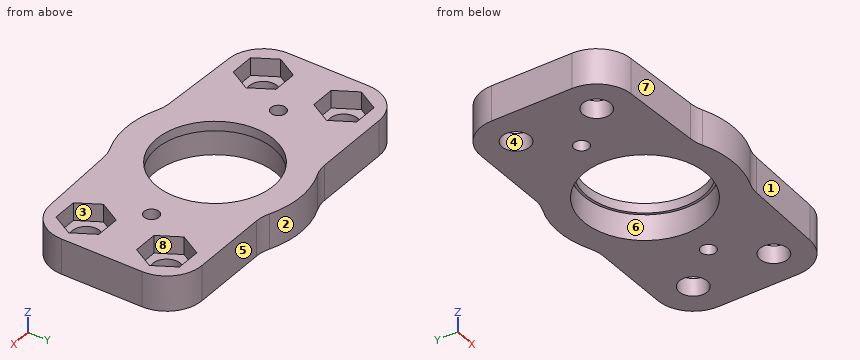
```python
from build123d import *

# Parameters (mm, degrees)
SKETCH_1_R          = 12.1
EXTRUDE_1_DEPTH     = 7
FILLET_3_R          = 7
SKETCH_7_R          = 12.1
SKETCH_7_R_2        = 11.6
EXTRUDE_2_DEPTH     = 1.9
HOLE_WIZARD_M53_D   = 5.5
HOLE_WIZARD_M54_D   = 5.5
CUT_EXTRUDE_1_DEPTH = 3.5
SKETCH1_R           = 1.475614807
CUT_EXTRUDE1_DEPTH  = 10


with BuildPart() as part:
    # Эскиз1 → Бобышка-Вытянуть1 (new body)
    with BuildSketch(Plane.XY):
        with BuildLine():
            Line((-9.282257481, -15.602398743), (-25.265839773, -14.994950265))
            ThreePointArc((-25.265839773, -14.994950265), (-30.042860221, -12.854849204), (-32, -8))
            Line((-32, -8), (-32, 15))
            Line((-32, 15), (-8, 15))
            ThreePointArc((-8, 15), (0, 17), (8, 15))
            Line((8, 15), (32, 15))
            Line((32, 15), (32, -8))
            ThreePointArc((32, -8), (30.042860221, -12.854849204), (25.265839773, -14.994950265))
            Line((25.265839773, -14.994950265), (9.282257481, -15.602398743))
            ThreePointArc((9.282257481, -15.602398743), (7.964469385, -15.770214084), (6.696960066, -16.167891819))
            ThreePointArc((6.696960066, -16.167891819), (0, -17.5), (-6.696960066, -16.167891819))
            ThreePointArc((-6.696960066, -16.167891819), (-7.964469385, -15.770214084), (-9.282257481, -15.602398743))
        make_face()
        Circle(SKETCH_1_R, mode=Mode.SUBTRACT)
    extrude(amount=EXTRUDE_1_DEPTH)

    # Скругление3
    fillet_3_edges = [part.edges().sort_by_distance(p)[0] for p in [
        (-32, 15, 3.5),
        (-8, 15, 3.5),
        (8, 15, 3.5),
        (32, 15, 3.5),
    ]]
    fillet(fillet_3_edges, radius=FILLET_3_R)

    # Эскиз7 → Бобышка-Вытянуть2 (add)
    with BuildSketch(Plane.XY.offset(7)):
        Circle(SKETCH_7_R)
        Circle(SKETCH_7_R_2, mode=Mode.SUBTRACT)
    extrude(amount=-EXTRUDE_2_DEPTH)

    # Отверстие с зазором M53 (through all)
    with Locations(Plane.XY.offset(7)):
        with Locations((-25, 8), (25, 8)):
            Hole(HOLE_WIZARD_M53_D / 2)

    # Отверстие с зазором M54 (through all)
    with Locations(Plane(origin=(-20.850360387, 7.199740636, 7), x_dir=(-1, 0, 0), z_dir=(0, 0, 1))):
        with Locations((-45.850360387, 15.199740636), (4.149639613, 15.199740636)):
            Hole(HOLE_WIZARD_M54_D / 2)

    # Эскиз18 → Вырез-Вытянуть1 (cut)
    with BuildSketch(Plane(origin=(0, 0, 7), x_dir=(1, 0, 0), z_dir=(0, 0, -1))):
        Polygon((20.092522712, -8), (22.546261356, -12.25), (27.453738644, -12.25), (29.907477288, -8), (27.453738644, -3.75), (22.546261356, -3.75), align=None)
        Polygon((-27.453738644, -3.75), (-29.907477288, -8), (-27.453738644, -12.25), (-22.546261356, -12.25), (-20.092522712, -8), (-22.546261356, -3.75), align=None)
        Polygon((20.092522712, 8), (22.546261356, 12.25), (27.453738644, 12.25), (29.907477288, 8), (27.453738644, 3.75), (22.546261356, 3.75), align=None)
        Polygon((-22.546261356, 12.25), (-20.092522712, 8), (-22.546261356, 3.75), (-27.453738644, 3.75), (-29.907477288, 8), (-27.453738644, 12.25), align=None)
    extrude(amount=CUT_EXTRUDE_1_DEPTH, mode=Mode.SUBTRACT)

    # Sketch1 → Cut-Extrude1 (cut)
    with BuildSketch(Plane.XY):
        with Locations((17.9, 0)):
            Circle(SKETCH1_R)
        with Locations((-17.9, 0)):
            Circle(SKETCH1_R)
    extrude(amount=CUT_EXTRUDE1_DEPTH, mode=Mode.SUBTRACT)


solid = part.part
```
Verification items for the finished model (mm, model axes). Face numbers are marked on the shaded views. A direction names the side the tool comes from. Coordinates: 2 decimals unless noted, no trailing zeros. Order: outer loops, then holes, each group sorted by start corner. A loop starts at its lowest first (then second) coordinate and runs counter-clockwise, first axis right, second up. Notation, with made-up numbers: (51, 42) -> (75, 42) arc R36 cw to (75, 81) -> close; hole circle Ø3 at (35.25, 58.25). An arc over 180 degrees is marked (long way). Answer as CSV lines item,"result". Start each with the question number.
1) Cross-section at C-C, the plane z = 1.75. Record the boundary of the cut face in (x, y), then the cut area to 3 significant figures.
2) Cross-section at B-B, the plane x = 0. Record the boundary of the cut face in (y, z).
3) Release check for a two-part mould opening along X. For the marked faces 1, 2, 3 and 4 record: released by +X, released by -X, zero draft, split by the parting line, or undercut.
4) Cross-section at A-A, the plane y = 0. Record the boundary of the cut face in (x, z).
5) Gauge pin test, flat ends, axial feed: pin 1 Ø4 at (x, y) = (25.5, -9) entering from +Z; pin 2 Ø2 at (x, z) = (-24.5, 1) entering from +Y; pin 3 Ø5 at (x, y) = (-25, -8) entering from -Z; pin 4 Ø1 at (x, z) = (26, 5) entering from -Y. Record the tip position at first contact, or that the pin passes through.
6) Cross-section at D-D, the plane x = 11. Record the boundary of the cut face in (y, z).
7) Material ranges on L1, parallel to Y at x = 24, z = 1.25; L2, parallel to Y at x = -25, z = 1.2; L3, parallel to X at y = -8.5, z = 2.5, recorded low to high. Write a range as [from, to].
8) Set-up check for the marked faces 5, 6, 7 and 8: record each of +Z, -Z, +X, -X, +Y, -Y from which the full face is reachable in a straight line by a thin tool's end or side.
Conclusion:
1,outline,"(-32, -8) arc R7 ccw to (-25.27, -14.99) -> (-9.28, -15.6) arc R7.5 cw to (-6.7, -16.17) arc R17.5 ccw to (6.7, -16.17) arc R7.5 cw to (9.28, -15.6) -> (25.27, -14.99) arc R7 ccw to (32, -8) -> (32, 8) arc R7 ccw to (25, 15) -> (9.59, 15) arc R7 cw to (6.79, 15.58) arc R17 ccw to (-6.79, 15.58) arc R7 cw to (-9.59, 15) -> (-25, 15) arc R7 ccw to (-32, 8) -> close; hole circle Ø5.5 at (-25, -8); hole circle Ø5.5 at (-25, 8); hole circle Ø2.95 at (-17.9, 0); hole circle Ø24.2 at (0, 0); hole circle Ø2.95 at (17.9, 0); hole circle Ø5.5 at (25, -8); hole circle Ø5.5 at (25, 8)"
1,area,"1,370 mm²"
2,outline,"(-17.5, 0) -> (-12.1, 0) -> (-12.1, 5.1) -> (-11.6, 5.1) -> (-11.6, 7) -> (-17.5, 7) -> close; (11.6, 5.1) -> (12.1, 5.1) -> (12.1, 0) -> (17, 0) -> (17, 7) -> (11.6, 7) -> close"
3,face 1,"released by +X"
3,face 2,"split by the parting line"
3,face 3,"undercut"
3,face 4,"undercut"
4,outline,"(-32, 0) -> (-19.38, 0) -> (-19.38, 7) -> (-32, 7) -> close; (-16.42, 0) -> (-12.1, 0) -> (-12.1, 5.1) -> (-11.6, 5.1) -> (-11.6, 7) -> (-16.42, 7) -> close; (11.6, 5.1) -> (12.1, 5.1) -> (12.1, 0) -> (16.42, 0) -> (16.42, 7) -> (11.6, 7) -> close; (19.38, 0) -> (32, 0) -> (32, 7) -> (19.38, 7) -> close"
5,pin 1,"stops at z = 3.5"
5,pin 2,"stops at y = 15"
5,pin 3,"passes through"
5,pin 4,"stops at y = -14.98"
6,outline,"(-15.54, 0) -> (-5.04, 0) -> (-5.04, 5.1) -> (-3.68, 5.1) -> (-3.68, 7) -> (-15.54, 7) -> close; (3.68, 5.1) -> (5.04, 5.1) -> (5.04, 0) -> (15, 0) -> (15, 7) -> (3.68, 7) -> close"
7,L1,"y = [-15.04, -10.56], [-5.44, 5.44], [10.56, 15]"
7,L2,"y = [-15.01, -10.75], [-5.25, 5.25], [10.75, 15]"
7,L3,"x = [-31.98, -27.7], [-22.3, -8.61], [8.61, 22.3], [27.7, 31.98]"
8,face 5,"+Z, -Z, +X, +Y"
8,face 6,"-Z"
8,face 7,"+Z, -Z, -X, -Y"
8,face 8,"+Z"
